from build123d import *

# Parameters (mm, degrees)
BOSS_EXTRUDE1_DEPTH = 5
SKETCH2_W           = 30
SKETCH2_H           = 5
CUT_EXTRUDE1_DEPTH  = 5
CUT_EXTRUDE2_DEPTH  = 5
BOSS_EXTRUDE2_START = 15
BOSS_EXTRUDE2_DEPTH = 5
BOSS_EXTRUDE3_START = 5
BOSS_EXTRUDE3_DEPTH = 5
CUT_EXTRUDE3_DEPTH  = 10


with BuildPart() as part:
    # Sketch1 → Boss-Extrude1 (new body)
    with BuildSketch(Plane(origin=(0, 0, 0), x_dir=(1, 0, 0), z_dir=(0, 1, 0))):
        Polygon((-53.033008589, 0), (53.033008589, 0), (0, 53.033008589), align=None)
    extrude(amount=BOSS_EXTRUDE1_DEPTH)

    # Sketch2 → Cut-Extrude1 (cut)
    with BuildSketch(Plane(origin=(0, 5, 0), x_dir=(1, 0, 0), z_dir=(0, 1, 0))):
        with Locations((0, 2.5)):
            Rectangle(SKETCH2_W, SKETCH2_H)
        Polygon((-3.535533906, 49.497474683), (-24.748737342, 28.284271247), (-21.213203436, 24.748737342), (0, 45.961940777), align=None)
    extrude(amount=-CUT_EXTRUDE1_DEPTH, mode=Mode.SUBTRACT)

    # Sketch3 → Cut-Extrude2 (cut)
    with BuildSketch(Plane.XZ):
        Polygon((15.909902577, -37.123106012), (37.123106012, -15.909902577), (33.587572106, -12.374368671), (12.374368671, -33.587572106), align=None)
    extrude(amount=-CUT_EXTRUDE2_DEPTH, mode=Mode.SUBTRACT)

    # Sketch5 → Boss-Extrude2 (add)
    with BuildSketch(Plane.ZY.offset(-15).offset(BOSS_EXTRUDE2_START)):
        with BuildLine():
            Line((-2.5, 5), (-5, 5))
            ThreePointArc((-5, 5), (-3.535533906, 1.464466094), (0, 0))
            Line((0, 0), (0, 2.5))
            ThreePointArc((0, 2.5), (-1.767766953, 3.232233047), (-2.5, 5))
        make_face()
        with BuildLine():
            ThreePointArc((0, 0), (3.535533906, 1.464466094), (5, 5))
            ThreePointArc((5, 5), (0, 10), (-5, 5))
            Line((-5, 5), (-2.5, 5))
            ThreePointArc((-2.5, 5), (0, 7.5), (2.5, 5))
            ThreePointArc((2.5, 5), (1.767766953, 3.232233047), (0, 2.5))
            Line((0, 2.5), (0, 0))
        make_face()
        with BuildLine():
            ThreePointArc((0, 0), (-3.535533906, 1.464466094), (-5, 5))
            Line((-5, 5), (-5, 0))
            Line((-5, 0), (0, 0))
        make_face()
    extrude(amount=BOSS_EXTRUDE2_DEPTH)

    # Sketch6 → Boss-Extrude3 (add)
    with BuildSketch(Plane(origin=(10.606601718, 0, 10.606601718), x_dir=(-0.7071067811865478, 0, 0.7071067811865472), z_dir=(-0.7071067811865472, 0, -0.7071067811865478)).offset(BOSS_EXTRUDE3_START)):
        with BuildLine():
            ThreePointArc((-37.5, 5), (-41.035533906, -3.535533906), (-32.5, 0))
            Line((-32.5, 0), (-35, 0))
            ThreePointArc((-35, 0), (-39.267766953, -1.767766953), (-37.5, 2.5))
            Line((-37.5, 2.5), (-37.5, 5))
        make_face()
        with BuildLine():
            Line((-35, 0), (-32.5, 0))
            ThreePointArc((-32.5, 0), (-33.964466094, 3.535533906), (-37.5, 5))
            Line((-37.5, 5), (-37.5, 2.5))
            ThreePointArc((-37.5, 2.5), (-35.732233047, 1.767766953), (-35, 0))
        make_face()
        with BuildLine():
            ThreePointArc((-37.5, 5), (-33.964466094, 3.535533906), (-32.5, 0))
            Line((-32.5, 0), (-32.5, 5))
            Line((-32.5, 5), (-37.5, 5))
        make_face()
    extrude(amount=BOSS_EXTRUDE3_DEPTH)

    # Sketch7 → Cut-Extrude3 (cut)
    with BuildSketch(Plane.XZ):
        Polygon((-21.154129879, -31.87887871), (0, -53.033008589), (2.121320344, -50.911688245), (-19.032809536, -29.757558366), align=None)
    extrude(amount=-CUT_EXTRUDE3_DEPTH, mode=Mode.SUBTRACT)


solid = part.part
Geometry check sheet. Reference: the model listing, model coordinates, mm. A direction names the side the tool comes from. Round coordinates to 2 decimals unless told otherwise and drop trailing zeros. Loops run counter-clockwise (first coordinate to the right, second up) from the corner with the lowest first, then second, coordinate; pieces in that order, holes last. Notation, with made-up numbers: (-31.5, 59) - (20.5, 59) arc R16 ccw to (20.5, 78) - close; hole circle Ø2 at (48, 43). An arc over 180 degrees is marked (long way). One line per question, with ' | ' between items. Start each with the question number.
1. Draft check along X on faces 5 (the face through (0.38, 2.46, -49.17)), 6 (the face through (-1, 5, -14)), 7 (the face through (19.54, 2.46, -26.42)). Enter one of: released by +X, released by -X, zero draft, split by the parting line, or undercut.
2. Cross-section at C-C on z = -35. Record the cut outline in (x, y), then the cut area to 3 significant figures.
3. Cross-section at A-A on y = 3.5. Record the cut outline in (x, z), then the cut area to 3 significant figures.
4. Depth check by flat-ended pin: pin 1 (4 mm diameter, centred on x = 40, y = 4, fed in from -Z); pin 2 (3 mm diameter, centred on y = 0, z = -34, fed in from -X); pin 3 (2.5 mm diameter, centred on x = 37.5, y = 2, fed in from +Z); pin 4 (3 mm diameter, centred on x = 5.5, y = -3, fed in from -Z). Enter the tip coordinate at first touch or a pass-through.
5. Cross-section at B-B on x = -4. Record the cut outline in (y, z), then the cut area to 3 significant figures.
6. Tool access check on faces 1 (the face through (14.117, 2.465, -35.331)), 2 (the face through (34, 2, 0)), 3 (the face through (28.53, 2.29, -21.46)), 4 (the face through (7, 3, -5)). Record the directions out of +Z, -Z, +X, -X, +Y, -Y that give a thin tool (end or side, any length) a straight path to the whole face; none if there is none.
7. Scan lines: line 1 (Y direction, x = -16, z = -18); line 2 (X direction, y = 5.5, z = 2.5); line 3 (Z direction, x = -2, y = 7). Record each from-to range of solid material in increasing order. Write a range as [from, to].
8. Cross-section at D-D on x = 38.5. Record the cut outline in (y, z), then the cut area to 3 significant figures.
Taken from the geometry:
1) face 5: released by -X | face 6: zero draft | face 7: undercut
2) outline: (-10.96, 0) - (13.79, 0) - (13.79, 5) - (-10.96, 5) - close | area: 124 mm²
3) outline: (-53.03, 0) - (-24.75, -28.28) - (-21.21, -24.75) - (0, -45.96) - (-1.41, -47.38) - (2.12, -50.91) - (15.91, -37.12) - (12.37, -33.59) - (26.52, -19.45) - (32.58, -25.51) - (36.11, -21.97) - (30.05, -15.91) - (33.59, -12.37) - (37.12, -15.91) - (53.03, 0) - (15, 0) - (15, -5) - (0, -5) - (0, -2) - (-5, -2) - (-5, -5) - (-15, -5) - (-15, 0) - close; (-5, 2) - (0, 2) - (0, 4.77) - (-5, 4.77) - close | area: 2,420 mm²
4) pin 1: z = -15.03 | pin 2: x = -13.46 | pin 3: z = 0 | pin 4: through
5) outline: (0, -41.96) - (5, -41.96) - (5, -5) arc R5 ccw (long way) to (0, 0) - close; hole circle Ø5 at (5, 0) | area: 249 mm²
6) face 1: +X, +Y, -Y | face 2: +Z, +X, +Y, -Y | face 3: -Z, +Y, -Y | face 4: +Z, +Y, -Y
7) line 1: [0, 5] | line 2: [-5, 0] | line 3: [-4.58, -1.5], [1.5, 4.58]
8) outline: (0, -14.53) - (5, -14.53) - (5, 0) - (0, 0) - close | area: 72.7 mm²
